Can you work these out from the drawing? Everything is in mm from the part's minimum corner. A direction names the side the tool comes from. Give positions to 0.01 mm unless a question says otherwise; leave off trailing zeros. Loops run counter-clockwise (first coordinate to the right, second up) from the corner with the lowest first, then second, coordinate; pieces in that order, holes last. Notation, with made-up numbers: (83.25, 57.25) -> (112.25, 57.25) arc R25 cw to (112.25, 91.25) -> close; hole circle Ø4 at (-15.5, -24). An arc over 180 degrees is marked (long way). Return JSON: item names as keys, results as strings. Group by question number.
Q1. Suppose I cut it at A-A, the plane z = 7. Please give me the cut outline in (x, y), and give its area (3 significant figures).
Q2. I need wall thicknesses on line 1 along X through (y, z) = (1.65, 7); line 2 along Y through (x, z) = (13, 6.5); line 3 along X through (y, z) = (12.25, 3.5). Which ranges of each line are inside material? Lowest first, please. Write a range as [from, to].
Q3. Suppose I cut it at B-B, the plane x = 4.25. Please give me the cut outline in (y, z).
Q4. Which directions (+Z, -Z, +X, -X, +Y, -Y) give clear straight access to the entire face, cutting with the end or side of a thin tool? Please do the marked faces 4 and 5.
Q5. Will these pins go through, and if not, where does the flat tip stop? pin 1 (5 mm diameter, centred on x = 4, y = 7, fed in from -Z); pin 2 (1.5 mm diameter, centred on y = 4, z = 10, fed in from -X); pin 3 (2 mm diameter, centred on y = 5, z = 9.5, fed in from +X).
Q6. Suppose I cut it at C-C, the plane y = 8.5. Please give me the cut outline in (x, z), and give its area (3 significant figures).
Q7. Thinking about a two-plate mould opening in Z: for the marked faces 1, 2 and 3, which applies, pulls with the +Z half, pulls with the -Z half, needs draft (parallel to the pull), parting line crosses it, or undercut?
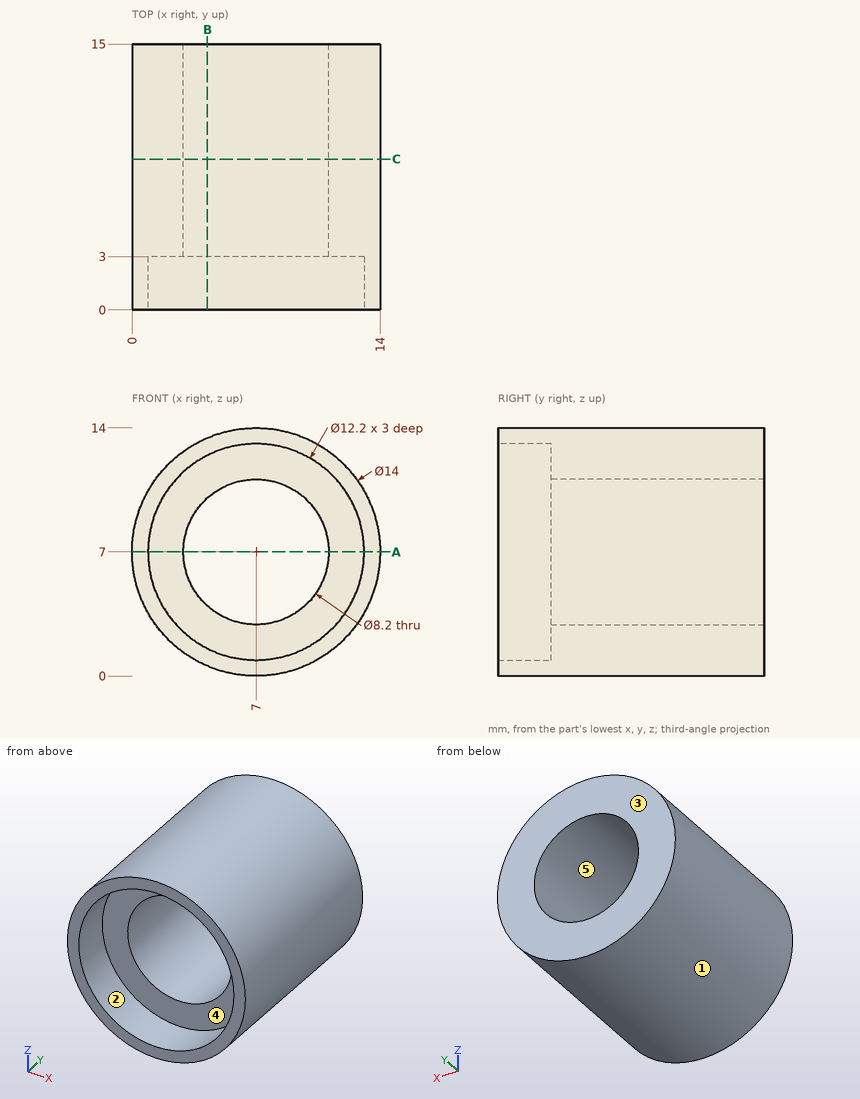
Ans:
{
 "1": {"outline": "(0, 0) -> (0.9, 0) -> (0.9, 3) -> (2.9, 3) -> (2.9, 15) -> (0, 15) -> close; (11.1, 3) -> (13.1, 3) -> (13.1, 0) -> (14, 0) -> (14, 15) -> (11.1, 15) -> close", "area": "75.0 mm^2"},
 "2": {"line 1": "x = [0, 0.9], [13.1, 14]", "line 2": "y = [3, 15]", "line 3": "x = [0.94, 4.86], [9.14, 13.06]"},
 "3": {"outline": "(0, 0.56) -> (15, 0.56) -> (15, 3.96) -> (3, 3.96) -> (3, 1.56) -> (0, 1.56) -> close; (0, 12.44) -> (3, 12.44) -> (3, 10.04) -> (15, 10.04) -> (15, 13.44) -> (0, 13.44) -> close"},
 "4": {"face 4": "-Y", "face 5": "+Y, -Y"},
 "5": {"pin 1": "stops at z = 0.02", "pin 2": "stops at x = 0.37", "pin 3": "stops at x = 13.84"},
 "6": {"outline": "circle Ø14 at (7, 7); hole circle Ø8.2 at (7, 7)", "area": "101 mm^2"},
 "7": {"face 1": "parting line crosses it", "face 2": "undercut", "face 3": "needs draft"}
}
